```python
from build123d import *

# Parameters (mm, degrees)
F1_DEPTH = 76.2


with BuildPart() as f1:
    # F0 (on Front) → F1 (new body)
    with BuildSketch(Plane.XZ):
        with BuildLine():
            ThreePointArc((-75, -34.5), (-74.12132, -36.62132), (-72, -37.5))
            Line((-72, -37.5), (72, -37.5))
            ThreePointArc((72, -37.5), (74.12132, -36.62132), (75, -34.5))
            Line((75, -34.5), (75, 34.5))
            ThreePointArc((75, 34.5), (74.12132, 36.62132), (72, 37.5))
            Line((72, 37.5), (43, 37.5))
            ThreePointArc((43, 37.5), (40.87868, 36.62132), (40, 34.5))
            Line((40, 34.5), (40, -4.5))
            ThreePointArc((40, -4.5), (39.12132, -6.62132), (37, -7.5))
            Line((37, -7.5), (-37, -7.5))
            ThreePointArc((-37, -7.5), (-39.12132, -6.62132), (-40, -4.5))
            Line((-40, -4.5), (-40, 34.5))
            ThreePointArc((-40, 34.5), (-40.87868, 36.62132), (-43, 37.5))
            Line((-43, 37.5), (-72, 37.5))
            ThreePointArc((-72, 37.5), (-74.12132, 36.62132), (-75, 34.5))
            Line((-75, 34.5), (-75, -34.5))
        make_face()
    extrude(amount=F1_DEPTH)


solid = f1.part
```
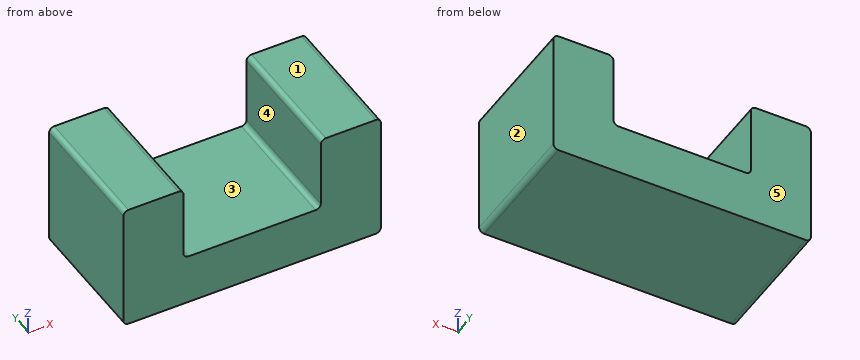
Part model, mm, in its own coordinate system. Face numbers are marked on the shaded views. A direction names the side the tool comes from. Round coordinates to 2 decimals unless told otherwise and drop trailing zeros. Loops run counter-clockwise (first coordinate to the right, second up) from the corner with the lowest first, then second, coordinate; pieces in that order, holes last. Notation, with made-up numbers: (47.5, 1.5) -> (91.5, 1.5) arc R17 ccw to (91.5, 21.5) -> close; hole circle Ø6 at (70, 25.5). An arc over 180 degrees is marked (long way). Use CSV: the item, a comma, the result in double quotes. Start each with the question number.
1) Cut at C-C, the plane x = -15. Write the cut outline in (y, z).
2) Pull direction X, two halves, no side cores. Call the marked faces 1, 2 and 3: +X half, -X half, draft (parallel to the pull), parting line (faces both ways), or undercut.
3) Which spindle directions (+Z, -Z, +X, -X, +Y, -Y) get a long thin tool onto all of the face, cutting with end or side? Do the marked faces 4 and 5. Say none if no direction does.
4) Cut at B-B, the plane y = -62.5. Write the cut outline in (x, z).
5) Drop a flat-ended pin along its axis: P1, Ø12, axis at x = 5, y = -46.5, coming from the +Z side. Give the stop position or say it passes through.
6) Cut at A-A, the plane z = 30. Write the cut outline in (x, y), plus the area to 3 significant figures.
7) Wall check: L1, parallel to X at y = -20.5, z = 15; L2, parallel to Z at x = -11.5, y = -4; L3, parallel to X at y = -10.5, z = -7. Give the ranges that are in metal, low to high. Write a range as [from, to].
Determined:
1,outline,"(-76.2, -37.5) -> (0, -37.5) -> (0, -7.5) -> (-76.2, -7.5) -> close"
2,face 1,"draft"
2,face 2,"+X half"
2,face 3,"undercut"
3,face 4,"+Z, +Y, -Y"
3,face 5,"+Z, -Z, +X, -X, +Y"
4,outline,"(-75, -34.5) arc R3 ccw to (-72, -37.5) -> (72, -37.5) arc R3 ccw to (75, -34.5) -> (75, 34.5) arc R3 ccw to (72, 37.5) -> (43, 37.5) arc R3 ccw to (40, 34.5) -> (40, -4.5) arc R3 cw to (37, -7.5) -> (-37, -7.5) arc R3 cw to (-40, -4.5) -> (-40, 34.5) arc R3 ccw to (-43, 37.5) -> (-72, 37.5) arc R3 ccw to (-75, 34.5) -> close"
5,P1,"stops at z = -7.5"
6,outline,"(-75, -76.2) -> (-40, -76.2) -> (-40, 0) -> (-75, 0) -> close; (40, -76.2) -> (75, -76.2) -> (75, 0) -> (40, 0) -> close"
6,area,"5,330 mm2"
7,L1,"x = [-75, -40], [40, 75]"
7,L2,"z = [-37.5, -7.5]"
7,L3,"x = [-75, -38.66], [38.66, 75]"
